```python
from build123d import *

# Parameters (mm, degrees)
EXTRUDE_1_DEPTH = 12
SKETCH_2_R      = 1.25
EXTRUDE_2_DEPTH = 6


# Read off the part's stored shape, not the designer's step: M3 螺纹孔1
with BuildPart() as part:
    # 草图1 → 凸台-拉伸1 (new body)
    with BuildSketch(Plane.XY):
        Polygon((2.598076211, 0), (1.299038106, 2.25), (-1.299038106, 2.25), (-2.598076211, 0), (-1.299038106, -2.25), (1.299038106, -2.25), align=None)
    extrude(amount=EXTRUDE_1_DEPTH)

    # 草图2 → 凸台-拉伸2 (add)
    with BuildSketch(Plane.XY.offset(12)):
        Circle(SKETCH_2_R)
    extrude(amount=EXTRUDE_2_DEPTH)

    # M3 螺纹孔1 outline → M3 螺纹孔1 (revolve, cut)
    with BuildSketch(Plane.XZ):
        Polygon((1.25, 7.5), (0, 8.251075774), (0, 0), (1.25, 0), align=None)
    revolve(axis=Axis((0, 0, 0), (0, 0, 1)), mode=Mode.SUBTRACT)


solid = part.part
```
Design review of the part built by this model. Coordinates are the model's own, in mm. A direction names the side the tool comes from. Give positions to 0.01 mm unless a question says otherwise; leave off trailing zeros. Write each loop counter-clockwise with the first axis right and the second up, starting at its lowest first coordinate (ties: lowest second). Pieces come first, ordered by that corner, then holes. Notation, with made-up numbers: (-24.5, 65) -> (15.5, 65) arc R18 ccw to (15.5, 79) -> close; hole circle Ø11 at (43, 87). An arc over 180 degrees is marked (long way). Answer in a Markdown table with one row per item.
(1) For faces 1 (the flat face through (-1.94, 1.14, 5.92)), 2 (the flat face through (-1, 1, 12)), list the 3-axis set-ups (+Z, -Z, +X, -X, +Y, -Y) from which the entire face can be reached by the end or side of a thin tool; tool diameter is ignored.
Results:
| item | result |
|---|---|
| face 1 | +Z, -Z, -X, +Y |
| face 2 | +Z |
(2) Consider section A-A (z = 6.5). State the section outline as (x, y) points.
Results:
| item | result |
|---|---|
| outline | (-2.6, 0) -> (-1.3, -2.25) -> (1.3, -2.25) -> (2.6, 0) -> (1.3, 2.25) -> (-1.3, 2.25) -> close; hole circle Ø2.5 at (0, 0) |
(3) Consider section B-B (z = 12.25). State the section outline as (x, y) points, then the cut area to 3 significant figures.
Results:
| item | result |
|---|---|
| outline | circle Ø2.5 at (0, 0) |
| area | 4.91 mm2 |
(4) To check wall thickness, follow probe 1 along Y at (x, z) = (0, 2.25); probe 2 along X at (y, z) = (-0.75, 2.5); probe 3 along Z at (x, y) = (1.35, 1.35). State the ranges of each line that lie inside material, in increasing order.
Results:
| item | result |
|---|---|
| probe 1 | -2.25 to -1.25, 1.25 to 2.25 |
| probe 2 | -2.17 to -1, 1 to 2.17 |
| probe 3 | 0 to 12 |
(5) Consider section C-C (x = -1.85). State the section outline as (y, z) points.
Results:
| item | result |
|---|---|
| outline | (-1.3, 0) -> (1.3, 0) -> (1.3, 12) -> (-1.3, 12) -> close |
(6) Mouldability with a two-part tool opening along Y and no side actions: class faces 3 (the cylindrical face through (-0.27, -1.22, 3.8)), 4 (the flat face through (1.94, -1.14, 5.92)), 5 (the flat face through (-1, 1, 0)) as +Y half, -Y half, draft (parallel to the pull), parting line (faces both ways), or undercut.
Results:
| item | result |
|---|---|
| face 3 | undercut |
| face 4 | -Y half |
| face 5 | draft |
(7) Consider section D-D (y = -1.85). State the section outline as (x, z) points.
Results:
| item | result |
|---|---|
| outline | (-1.53, 0) -> (1.53, 0) -> (1.53, 12) -> (-1.53, 12) -> close |
